Verification items for the finished model (mm, model axes). Round coordinates to 2 decimals unless told otherwise and drop trailing zeros. Write each loop counter-clockwise with the first axis right and the second up, starting at its lowest first coordinate (ties: lowest second). Pieces come first, ordered by that corner, then holes.
from build123d import *

# Parameters (mm, degrees)
F0_W     = 25
F0_H     = 25
F1_DEPTH = 5
F3_DEPTH = 12
F4_DEPTH = 5.001


with BuildPart() as f1:
    # F0 (on Top) → F1 (new body)
    with BuildSketch(Plane.XY):
        with Locations((-12.5, 12.5)):
            Rectangle(F0_W, F0_H)
        Polygon((25, 25), (0, 25), (0, 0), (-25, 0), (-25, -25), (25, -25), align=None)
    extrude(amount=F1_DEPTH)

    # F2 (on face) → F3 (join)
    with BuildSketch(Plane.XY.offset(5)):
        with BuildLine():
            ThreePointArc((18.7736850405, -18.7736850405), (19.5685222451, -22.7696015091), (22.9560966544, -20.5060966544))
            ThreePointArc((22.9560966544, -20.5060966544), (21.4436710637, -18.2425917998), (18.7736850405, -18.7736850405))
        make_face()
    extrude(amount=F3_DEPTH)

    # F2 (on face) → F4 (cut, through all)
    with BuildSketch(Plane.XY.offset(5)):
        with BuildLine():
            ThreePointArc((-17.9560966544, 20.5060966544), (-22.8619894623, 21.4819394069), (-18.7029743624, 18.7029743624))
            ThreePointArc((-18.7029743624, 18.7029743624), (-18.1502038465, 19.5302539019), (-17.9560966544, 20.5060966544))
        make_face()
    extrude(amount=-F4_DEPTH, mode=Mode.SUBTRACT)


solid = f1.part
Q1. Depth check by flat-ended pin: P1, Ø15, axis at x = 8, y = 8.5, coming from the +Z side. Enter the tip coordinate at first touch or a pass-through.
Recorded:
P1: stops at z = 5
Q2. Sectioned sample at C-C (z = 15.5). Enter the section's corners in (x, y), plus the area to 3 significant figures.
Recorded:
outline: circle Ø4.9 at (20.51, -20.51)
area: 18.9 mm2
Q3. Sectioned sample at B-B (y = -13.5). Enter the section's corners in (x, z).
Recorded:
outline: (-25, 0) - (25, 0) - (25, 5) - (-25, 5) - close
Q4. Sectioned sample at A-A (x = -21). Enter the section's corners in (y, z), plus the area to 3 significant figures.
Recorded:
outline: (-25, 0) - (18, 0) - (18, 5) - (-25, 5) - close; (23.01, 0) - (25, 0) - (25, 5) - (23.01, 5) - close
area: 225 mm2
Q5. Material ranges on line 1 along Z through (x, y) = (-19, 6); line 2 along X through (y, z) = (19, 1.75); line 3 along Y through (x, z) = (20.5, 5.5), recorded low to high.
Recorded:
line 1: z = 0 to 5
line 2: x = -25 to -22.56, -18.45 to 25
line 3: y = -22.96 to -18.06
